Design review of the part built by this model. Coordinates are the model's own, in mm. Face numbers are marked on the shaded views. A direction names the side the tool comes from. Coordinates: 2 decimals unless noted, no trailing zeros. Write each loop counter-clockwise with the first axis right and the second up, starting at its lowest first coordinate (ties: lowest second). Pieces come first, ordered by that corner, then holes. Notation, with made-up numbers: (-27, 56.5) -> (11, 56.5) arc R21 ccw to (11, 63.5) -> close; hole circle Ø11 at (78.25, 16). An arc over 180 degrees is marked (long way). Write item = value, one per line. Start each with the question number.
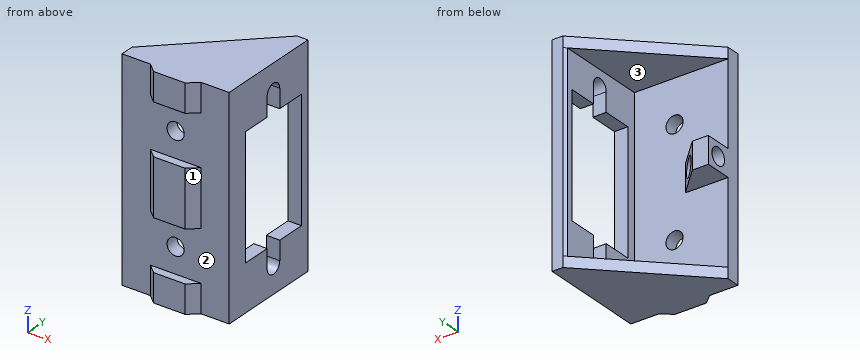
```python
from build123d import *

# Parameters (mm, degrees)
PAD_DEPTH            = 40
PAD001_DEPTH         = 40
SKETCH002_W          = 17.5
SKETCH002_H          = 36
POCKET_DEPTH         = 18
SKETCH003_W          = 14.2
SKETCH003_H          = 22.7
POCKET001_DEPTH      = 2.001
SKETCH004_R          = 1.6
POCKET002_DEPTH      = 21.561
SKETCH005_W          = 9.48
SKETCH005_H          = 9.48
POCKET003_DEPTH      = 1.56
POCKET003_FACE12_W   = 17.5
POCKET003_FACE12_H   = 36
POCKET003_FACE12_W_2 = 14.2
POCKET003_FACE12_H_2 = 22.7
PAD002_DEPTH         = 0.5
POCKET004_DEPTH      = 38.001
POCKET005_DEPTH      = 2.5
SKETCH007_W          = 3
SKETCH007_H          = 5
PAD003_DEPTH         = 5
CHAMFER_SIZE         = 4.99
SKETCH008_R          = 1.6
POCKET006_DEPTH      = 17.5


with BuildPart() as part:
    # Sketch → Pad (new body)
    with BuildSketch(Plane.XY):
        Polygon((-10, -8.75), (-10, -11.25), (-4.74, -11.25), (-2.94, -12.81), (2.94, -12.81), (4.74, -11.25), (10, -11.25), (10, 8.75), (8, 8.75), (8, -8.75), align=None)
    extrude(amount=PAD_DEPTH)

    # Sketch001 (on Face11 of Pad) → Pad001 (join)
    with BuildSketch(Plane(origin=(0, 0, 0), x_dir=(1, 0, 0), z_dir=(0, 0, -1))):
        Polygon((-10, 8.75), (8, -8.75), (8, 8.75), align=None)
    extrude(amount=-PAD001_DEPTH)

    # Sketch002 (on Face1 of Pad001) → Pocket (cut)
    with BuildSketch(Plane(origin=(-10, 0, 0), x_dir=(0, -1, 0), z_dir=(-1, 0, 0))):
        with Locations((0, 20)):
            Rectangle(SKETCH002_W, SKETCH002_H)
    extrude(amount=-POCKET_DEPTH, mode=Mode.SUBTRACT)

    # Sketch003 (on Face12 of Pocket) → Pocket001 (cut, through all)
    with BuildSketch(Plane(origin=(8, 0, 0), x_dir=(0, -1, 0), z_dir=(-1, 0, 0))):
        with Locations((0, 20)):
            Rectangle(SKETCH003_W, SKETCH003_H)
    extrude(amount=-POCKET001_DEPTH, mode=Mode.SUBTRACT)

    # Sketch004 (on Face15 of Pocket001) → Pocket002 (cut, through all)
    with BuildSketch(Plane.XZ.offset(12.81)):
        with Locations((0, 30)):
            Circle(SKETCH004_R)
        with Locations((0, 10)):
            Circle(SKETCH004_R)
    extrude(amount=-POCKET002_DEPTH, mode=Mode.SUBTRACT)

    # Sketch005 (on Face17 of Pocket002) → Pocket003 (cut)
    with BuildSketch(Plane.XZ.offset(12.81)):
        with Locations((0, 30)):
            Rectangle(SKETCH005_W, SKETCH005_H)
        with Locations((0, 10)):
            Rectangle(SKETCH005_W, SKETCH005_H)
    extrude(amount=-POCKET003_DEPTH, mode=Mode.SUBTRACT)

    # Pocket003 Face12 → Pad002 (add)
    with BuildSketch(Plane(origin=(8, 0, 20), x_dir=(0, 1, 0), z_dir=(-1, 0, 0))):
        Rectangle(POCKET003_FACE12_W, POCKET003_FACE12_H)
        Rectangle(POCKET003_FACE12_W_2, POCKET003_FACE12_H_2, mode=Mode.SUBTRACT)
    extrude(amount=PAD002_DEPTH)

    # Pad002 Face11 → Pocket004 (cut, through all)
    with BuildSketch(Plane(origin=(7.666667, 8.587963, 2), x_dir=(0, -1, 0), z_dir=(0, 0, -1))):
        Polygon((-0.162037, -0.333333), (0.324074, 0.166667), (-0.162037, 0.166667), align=None)
    extrude(amount=-POCKET004_DEPTH, mode=Mode.SUBTRACT)

    # Sketch006 (on Face26 of Pocket004) → Pocket005 (cut)
    with BuildSketch(Plane.YZ.offset(10)):
        with BuildLine():
            ThreePointArc((1.6, 34.9), (0, 36.5), (-1.6, 34.9))
            Line((-1.6, 34.9), (-1.6, 5.1))
            ThreePointArc((-1.6, 5.1), (0, 3.5), (1.6, 5.1))
            Line((1.6, 5.1), (1.6, 34.9))
        make_face()
    extrude(amount=-POCKET005_DEPTH, mode=Mode.SUBTRACT)

    # Sketch007 (on Face3 of Pocket005) → Pad003 (join)
    with BuildSketch(Plane(origin=(0, -8.75, 0), x_dir=(-1, 0, 0), z_dir=(0, 1, 0))):
        with Locations((8.5, 20)):
            Rectangle(SKETCH007_W, SKETCH007_H)
    extrude(amount=PAD003_DEPTH)

    # Chamfer
    chamfer_edges = [part.edges().sort_by_distance(p)[0] for p in [
        (-7, -8.75, 20),
    ]]
    chamfer(chamfer_edges, length=CHAMFER_SIZE)

    # Sketch008 (on Face13 of Chamfer) → Pocket006 (cut)
    with BuildSketch(Plane(origin=(-10, 0, 0), x_dir=(0, -1, 0), z_dir=(-1, 0, 0))):
        with Locations((6.25, 20)):
            Circle(SKETCH008_R)
    extrude(amount=-POCKET006_DEPTH, mode=Mode.SUBTRACT)


solid = part.part
```
(1) Take a section at B-B, the plane x = 8.75. State the section outline as (y, z) points.
(2) For pin 1 Ø4 at (x, z) = (1, 33) entering from -Y; pin 2 Ø4 at (x, z) = (-8, 25.5) entering from +Y; pin 3 Ø1.2 at (x, z) = (9, 34) entering from -Y; pin 4 Ø10 at (x, z) = (-6.5, 25) entering from +Y, all flat-tipped, find the tip position at first contact; note any pin that passes through.
(3) Take a section at D-D, the plane z = 23. State the section outline as (x, y) points.
(4) Take a section at C-C, the plane z = 30. State the section outline as (x, y) points, then the cut area to 3 significant figures.
(5) For the marked faces 1, 2 and 3, list the 3-axis set-ups (+Z, -Z, +X, -X, +Y, -Y) from which the entire face can be reached by the end or side of a thin tool; tool diameter is ignored.
(6) For line 1 (Z direction, x = 0, y = -10.3); line 2 (Z direction, x = 5, y = 5.5); line 3 (Y direction, x = 8, z = 24.5), list the stretches that pass through material, from the lowest coordinate up.
(7) Take a section at A-A, the plane y = 0. State the section outline as (x, z) points, then the cut area to 3 significant figures.
Report:
q1.outline = (-11.25, 0) -> (8.75, 0) -> (8.75, 40) -> (-11.25, 40) -> close; hole (-7.1, 8.65) -> (-1.6, 8.65) -> (-1.6, 5.1) arc R1.6 ccw to (1.6, 5.1) -> (1.6, 8.65) -> (7.1, 8.65) -> (7.1, 31.35) -> (1.6, 31.35) -> (1.6, 34.9) arc R1.6 ccw to (-1.6, 34.9) -> (-1.6, 31.35) -> (-7.1, 31.35) -> close
q2.pin_1 = -12.81
q2.pin_2 = -8.75
q2.pin_3 = -11.25
q2.pin_4 = -3.75
q3.outline = (-10, -11.25) -> (-4.74, -11.25) -> (-2.94, -12.81) -> (2.94, -12.81) -> (4.74, -11.25) -> (10, -11.25) -> (10, -7.1) -> (7.5, -7.1) -> (7.5, -8.75) -> (-10, -8.75) -> close; (7.5, 7.1) -> (10, 7.1) -> (10, 8.75) -> (8, 8.75) -> (7.5, 8.26) -> close
q4.outline = (-10, -11.25) -> (-1.6, -11.25) -> (-1.6, -8.75) -> (-10, -8.75) -> close; (1.6, -11.25) -> (10, -11.25) -> (10, -7.1) -> (7.5, -7.1) -> (7.5, -8.75) -> (1.6, -8.75) -> close; (7.5, 7.1) -> (10, 7.1) -> (10, 8.75) -> (8, 8.75) -> (7.5, 8.26) -> close
q4.area = 50.1 mm2
q5.face_1 = +Z, -Z, +X, -Y
q5.face_2 = -Y
q5.face_3 = -X, +Y
q6.line_1 = 0 to 8.4, 11.6 to 28.4, 31.6 to 40
q6.line_2 = 0 to 2, 38 to 40
q6.line_3 = -11.25 to -7.1, 7.1 to 8.75
q7.outline = (-1, 0) -> (10, 0) -> (10, 3.5) -> (7.5, 3.5) -> (7.5, 2) -> (-1, 2) -> close; (-1, 38) -> (7.5, 38) -> (7.5, 36.5) -> (10, 36.5) -> (10, 40) -> (-1, 40) -> close
q7.area = 51.5 mm2
